Autodesk Inventor part; units mm, degrees
ref_plane "YZ Plane" through (0, 0, 0) normal (1, 0, 0) x (0, 1, 0)
ref_plane "XZ Plane" through (0, 0, 0) normal (0, 1, 0) x (-1, 0, 0)
ref_plane "XY Plane" through (0, 0, 0) normal (0, 0, 1) x (1, 0, 0)
sketch "Sketch1" plane through (0, 0, 0) normal (0, 0, 1) x (1, 0, 0)
  line L0 (-45.4918, 50) -> (54.5082, 50)
  line L1 (54.5082, 50) -> (54.5082, -50)
  line L2 (54.5082, -50) -> (-45.4918, -50)
  line L3 (-45.4918, -50) -> (-45.4918, 50)
  point P0 (0, 0)
  dimension "d0" = 100
  dimension "d1" = 100
extrude "Extrusion1" add sketch "Sketch1" along normal blind 20
sketch "Sketch2" plane through (0, 0, 20) normal (0, 0, 1) x (1, 0, 0)
  line L0 (-20.4918, 25) -> (29.5082, 25)
  line L1 (29.5082, 25) -> (29.5082, -25)
  line L2 (29.5082, -25) -> (-20.4918, -25)
  line L3 (-20.4918, -25) -> (-20.4918, 25)
  line L4 (54.5082, 50) -> (-45.4918, 50)
  line L5 (-45.4918, 50) -> (-45.4918, -50)
  line L6 (-45.4918, -50) -> (54.5082, -50)
  line L7 (54.5082, -50) -> (54.5082, 50)
  point P0 (0, 0)
  dimension "d4" = 25
  dimension "d5" = 25
  dimension "d6" = 25
  dimension "d7" = 25
extrude "Extrusion2" add sketch "Sketch2" along normal blind 120 contours L0 L1 L2 L3
sketch "Sketch3" plane through (29.5082, -25, 20) normal (1, 0, 0) x (0, 0, -1)
  line L0 (-120, 50) -> (-120, 0)
  circle A0 centre (-120, 25) radius 6
  point P0 (20, 25)
  dimension "d10" = 12
extrude "Extrusion3" cut sketch "Sketch3" against normal blind 50
sketch "Sketch4" plane through (0, 0, 140) normal (0, 0, 1) x (1, 0, 0)
  line L0 (19.5082, -11) -> (-10.4918, -11)
  line L1 (-10.4918, -11) -> (-10.4918, -20)
  line L2 (-10.4918, -20) -> (19.5082, -20)
  line L3 (19.5082, -20) -> (19.5082, -11)
  line L4 (19.5082, 20) -> (-10.4918, 20)
  line L5 (-10.4918, 20) -> (-10.4918, 11)
  line L6 (-10.4918, 11) -> (19.5082, 11)
  line L7 (19.5082, 11) -> (19.5082, 20)
  line L8 (29.5082, 6) -> (29.5082, 25)
  line L9 (-20.4918, 25) -> (-20.4918, 6)
  line L10 (29.5082, 25) -> (-20.4918, 25)
  line L11 (-20.4918, 6) -> (29.5082, 6)
  line L12 (29.5082, -6) -> (-20.4918, -6)
  line L13 (-20.4918, -25) -> (29.5082, -25)
  point P0 (0, 0)
  dimension "d13" = 10
  dimension "d14" = 10
  dimension "d15" = 5
  dimension "d16" = 5
  dimension "d17" = 5
  dimension "d18" = 5
extrude "Extrusion4" cut sketch "Sketch4" against normal blind 20 contours L3 L2 L1 L0 | L7 L6 L5 L4
equation "\"d1\" = d0"
equation "\"d5\" = d4"
equation "\"d6\" = d4"
equation "\"d7\" = d4"
properties part number "laser bottom" material "Iron, Cast"
Verification items for the finished model (mm, model axes). A direction names the side the tool comes from. Give positions to 0.01 mm unless a question says otherwise; leave off trailing zeros. Write each loop counter-clockwise with the first axis right and the second up, starting at its lowest first coordinate (ties: lowest second). Pieces come first, ordered by that corner, then holes. Notation, with made-up numbers: (78.5, 17) - (107.5, 17) arc R19 ccw to (107.5, 52) - close; hole circle Ø1 at (40, -17). An arc over 180 degrees is marked (long way). Answer as CSV lines item,"result". Start each with the question number.
1. Depth check by flat-ended pin: pin 1 (16 mm diameter, centred on x = 3, z = 133, fed in from -Y); pin 2 (10 mm diameter, centred on y = -12, z = 34, fed in from +X); pin 3 (4 mm diameter, centred on x = -0.5, z = 74.5, fed in from +Y); pin 4 (10 mm diameter, centred on x = -34.5, y = -1.5, fed in from -Z). Enter the tip coordinate at first touch or a pass-through.
2. Draft check along X on faces 1 (the face through (5, -11, 130)), 2 (the face through (4, -9, 140)), 3 (the face through (29.508, 0, 79)). Enter one of: pulls with the +X half, pulls with the -X half, needs draft (parallel to the pull), parting line crosses it, or undercut.
3. Sectioned sample at D-D (z = 88.5). Record the boundary of the cut face in (x, y).
4. Sectioned sample at C-C (z = 122). Record the boundary of the cut face in (x, y).
5. Set-up check for faces 4 (the face through (4, -20, 130)), 5 (the face through (4, 25, 79)), 6 (the face through (5, -25, 79)): record each of +Z, -Z, +X, -X, +Y, -Y from which the full face is reachable in a straight line by a thin tool's end or side.
6. Sectioned sample at B-B (y = -17.5). Record the boundary of the cut face in (x, z).
7. Sectioned sample at A-A (x = -13.5). Record the boundary of the cut face in (y, z), then the cut area to 3 significant figures.
8. Thickness scan on line 1 (Y direction, x = 9, z = 122); line 2 (Z direction, x = -31.5, y = -19); line 3 (Z direction, x = 18, y = -18). Record the ranges inside material, lowest first.
Derived:
1,pin 1,"y = -25"
1,pin 2,"x = 29.51"
1,pin 3,"y = 25"
1,pin 4,"z = 0"
2,face 1,"undercut"
2,face 2,"needs draft"
2,face 3,"pulls with the +X half"
3,outline,"(-20.49, -25) - (29.51, -25) - (29.51, 25) - (-20.49, 25) - close"
4,outline,"(-20.49, -25) - (29.51, -25) - (29.51, 25) - (-20.49, 25) - close; hole (-10.49, -20) - (19.51, -20) - (19.51, -11) - (-10.49, -11) - close; hole (-10.49, 11) - (19.51, 11) - (19.51, 20) - (-10.49, 20) - close"
5,face 4,"+Z"
5,face 5,"+Z, +X, -X, +Y"
5,face 6,"+Z, +X, -X, -Y"
6,outline,"(-45.49, 0) - (54.51, 0) - (54.51, 20) - (29.51, 20) - (29.51, 140) - (19.51, 140) - (19.51, 120) - (-10.49, 120) - (-10.49, 140) - (-20.49, 140) - (-20.49, 20) - (-45.49, 20) - close"
7,outline,"(-50, 0) - (50, 0) - (50, 20) - (25, 20) - (25, 140) - (6, 140) arc R6 cw to (-6, 140) - (-25, 140) - (-25, 20) - (-50, 20) - close"
7,area,"7,940 mm²"
8,line 1,"-25 to -20, -11 to 11, 20 to 25"
8,line 2,"0 to 20"
8,line 3,"0 to 120"
